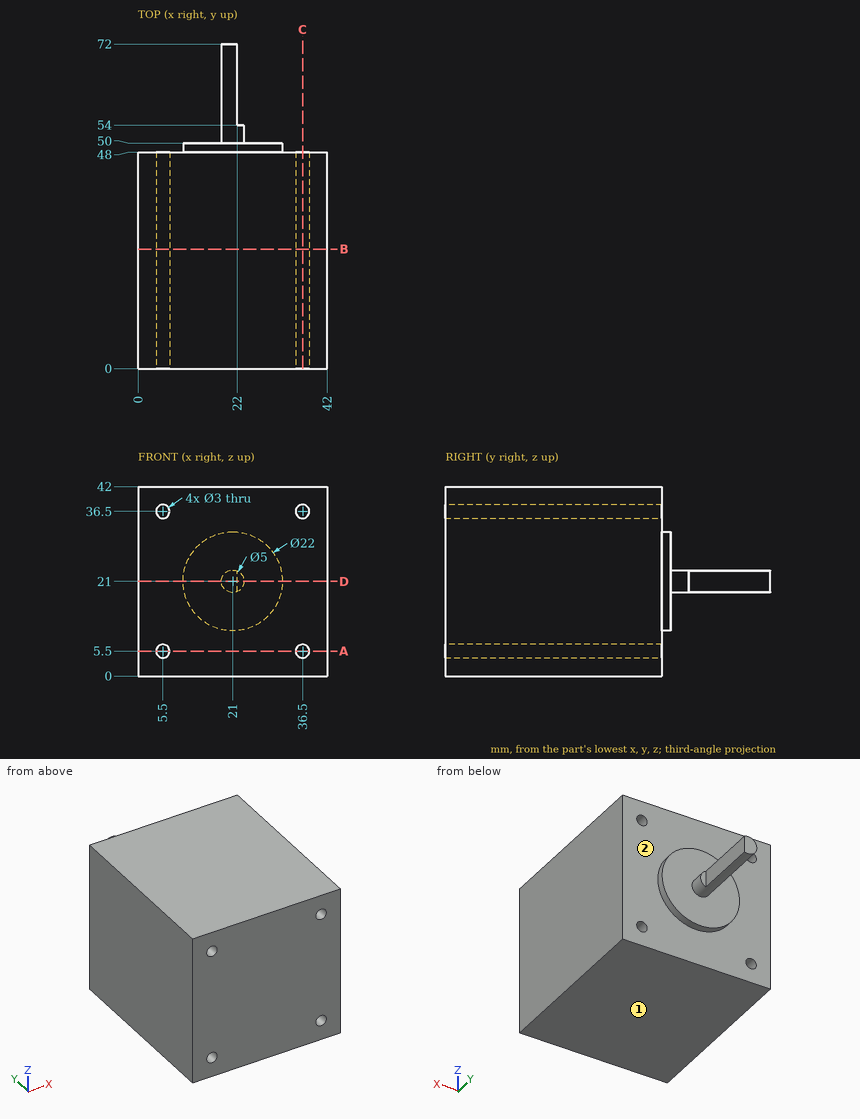
Part print with two shaded views. Sizes in mm from the minimum x, y, z corner. A direction names the side the tool comes from. Round coordinates to 2 decimals unless told otherwise and drop trailing zeros. Order: outer loops, then holes, each group sorted by start corner. A loop starts at its lowest first (then second) coordinate and runs counter-clockwise, first axis right, second up. Notation, with made-up numbers: M 22,4 L 63,4 A12 ccw 63,27 Z; hole C 74.5,53 d10. An arc over 180 degrees is marked long. Use CSV: the item, a comma, the result in double quotes.
Item 1: Saw through at C-C (x = 36.5). List the corners of the cut face in (y, z).
Worked answers:
outline,"M 0,0 L 48,0 L 48,4 L 0,4 Z; M 0,7 L 48,7 L 48,35 L 0,35 Z; M 0,38 L 48,38 L 48,42 L 0,42 Z"
Item 2: Pin check, flat tips, straight feed: pin 1 (1.2 mm diameter, centred on x = 22.5, z = 21.5, fed in from +Y); pin 2 (5 mm diameter, centred on y = 60.5, z = 22, fed in from +X); pin 3 (1.8 mm diameter, centred on x = 5.5, z = 5.5, fed in from +Y); pin 4 (3 mm diameter, centred on x = 23, z = 27, fed in from +Y). Stop position of each tip, or through.
Worked answers:
pin 1,"y = 72"
pin 2,"x = 22"
pin 3,"through"
pin 4,"y = 50"
Item 3: Probe probe 1 along X at (y, z) = (31, 36.5); probe 2 along X at (y, z) = (41, 4.5); probe 3 along Z at (x, y) = (6, 17). List the from-to ranges inside material, lowest first.
Worked answers:
probe 1,"0 to 4, 7 to 35, 38 to 42"
probe 2,"0 to 4.38, 6.62 to 35.38, 37.62 to 42"
probe 3,"0 to 4.09, 6.91 to 35.09, 37.91 to 42"
Item 4: Saw through at A-A (z = 5.5). List the corners of the cut face in (x, y).
Worked answers:
outline,"M 0,0 L 4,0 L 4,48 L 0,48 Z; M 7,0 L 35,0 L 35,48 L 7,48 Z; M 38,0 L 42,0 L 42,48 L 38,48 Z"
Item 5: Saw through at B-B (y = 26.5). List the corners of the cut face in (x, z).
Worked answers:
outline,"M 0,0 L 42,0 L 42,42 L 0,42 Z; hole C 5.5,5.5 d3; hole C 5.5,36.5 d3; hole C 36.5,5.5 d3; hole C 36.5,36.5 d3"
Item 6: Saw through at D-D (z = 21). List the corners of the cut face in (x, y), plus the area to 3 significant figures.
Worked answers:
outline,"M 0,0 L 42,0 L 42,48 L 32,48 L 32,50 L 23.5,50 L 23.5,54 L 22,54 L 22,72 L 18.5,72 L 18.5,50 L 10,50 L 10,48 L 0,48 Z"
area,"2,140 mm²"
Item 7: Which spindle directions (+Z, -Z, +X, -X, +Y, -Y) get a long thin tool onto all of the face, cutting with end or side? Do the marked faces 1 and 2. Say none if no direction does.
Worked answers:
face 1,"-Z, +X, -X, +Y, -Y"
face 2,"+Y"
